from build123d import *

# Parameters (mm, degrees)
SKETCH_2_W      = 70
SKETCH_2_H      = 20
SKETCH_2_R      = 2.6
EXTRUDE_1_DEPTH = 3
SKETCH_3_W      = 65
SKETCH_3_H      = 2
EXTRUDE_2_DEPTH = 10
FILLET_1_R      = 1
FILLET_2_R      = 5


with BuildPart() as part:
    # ｽｹｯﾁ2 → ﾎﾞｽ - 押し出し1 (new body)
    with BuildSketch(Plane.XY):
        Rectangle(SKETCH_2_W, SKETCH_2_H)
        with Locations((-25, 0)):
            Circle(SKETCH_2_R, mode=Mode.SUBTRACT)
        with Locations((25, 0)):
            Circle(SKETCH_2_R, mode=Mode.SUBTRACT)
        Circle(SKETCH_2_R, mode=Mode.SUBTRACT)
    extrude(amount=EXTRUDE_1_DEPTH)

    # ｽｹｯﾁ3 → ﾎﾞｽ - 押し出し2 (add)
    with BuildSketch(Plane.XY.offset(3)):
        with Locations((0, 9)):
            Rectangle(SKETCH_3_W, SKETCH_3_H)
    extrude(amount=EXTRUDE_2_DEPTH)

    # ﾌｨﾚｯﾄ1
    fillet_1_edges = [part.edges().sort_by_distance(p)[0] for p in [
        (-32.5, 10, 8),
        (-32.5, 8, 8),
        (32.5, 10, 8),
        (32.5, 8, 8),
    ]]
    fillet(fillet_1_edges, radius=FILLET_1_R - 0.0001)  # a hair under: the kernel refuses the full size

    # ﾌｨﾚｯﾄ2
    fillet_2_edges = [part.edges().sort_by_distance(p)[0] for p in [
        (-35, -10, 1.5),
        (-35, 10, 1.5),
        (35, -10, 1.5),
        (35, 10, 1.5),
    ]]
    fillet(fillet_2_edges, radius=FILLET_2_R)


solid = part.part
Input: part model. Units: mm. Frame: model coordinates. A direction names the side the tool comes from. Coordinates: 2 decimals unless noted, no trailing zeros. Order: outer loops, then holes, each group sorted by start corner. A loop starts at its lowest first (then second) coordinate and runs counter-clockwise, first axis right, second up. Notation, with made-up numbers: M 86.5,59 L 125.5,59 A13 ccw 125.5,83 Z; hole C 11.5,-7 d5. An arc over 180 degrees is marked long. Answer as CSV lines item,"result".
1. Access query for faces 5 (the flat face through (35, 0, 1)), 6 (the flat face through (0, 8, 8)). Directions: +Z, -Z, +X, -X, +Y, -Y. A direction counts if a zero-diameter tool reaches every point of the face in a straight line with its end or side. Return the directions, or none.
Reported:
face 5,"+Z, -Z, +X, +Y, -Y"
face 6,"+Z, +X, -X, -Y"
2. Pull-direction query (Y, two-part tool) for faces 1 (the flat face through (-35, 0, 1)), 2 (the cylindrical face through (-0.338, 2.578, 1.479)), 3 (the cylindrical face through (-22.52, 0.78, 1.48)), 4 (the cylindrical face through (-32.063, 9.554, 5.147)); classes: released by +Y, released by -Y, zero draft, split by the parting line, or undercut.
Reported:
face 1,"zero draft"
face 2,"undercut"
face 3,"undercut"
face 4,"released by +Y"
3. Material intervals for line 1 (Y direction, x = 0, z = 2.1); line 2 (X direction, y = 0.25, z = 1.5); line 3 (Y direction, x = 12, z = 9.5), sorted ascending. Write a range as from..to.
Reported:
line 1,"-10..-2.6, 2.6..10"
line 2,"-35..-27.59, -22.41..-2.59, 2.59..22.41, 27.59..35"
line 3,"8..10"
4. Section C-C (y = -2). Return the cut outline in (x, z).
Reported:
outline,"M -35,0 L -26.66,0 L -26.66,3 L -35,3 Z; M -23.34,0 L -1.66,0 L -1.66,3 L -23.34,3 Z; M 1.66,0 L 23.34,0 L 23.34,3 L 1.66,3 Z; M 26.66,0 L 35,0 L 35,3 L 26.66,3 Z"
5. Section A-A (x = -25). Return the cut outline in (y, z).
Reported:
outline,"M -10,0 L -2.6,0 L -2.6,3 L -10,3 Z; M 2.6,0 L 10,0 L 10,13 L 8,13 L 8,3 L 2.6,3 Z"
6. First-contact query: P1, Ø3, axis at y = 8, z = 3.5, coming from the -X side; P2, Ø9.5, axis at x = 3.5, y = -2.5, coming from the +Z side; P3, Ø1.5, axis at x = -22.5, z = 8.5, coming from the -Y side. Flat tips, straight axial feed; report the tip coordinate or a pass-through.
Reported:
P1,"x = -34.74"
P2,"z = 3"
P3,"y = 8"
7. Section B-B (x = 13.5). Return the cut outline in (y, z).
Reported:
outline,"M -10,0 L 10,0 L 10,13 L 8,13 L 8,3 L -10,3 Z"
